from build123d import *

# Parameters (mm, degrees)
F0_W = 19.05
F0_H = 38.1
F2_R = 6.35


with BuildPart() as f1:
    # F0 (on Front) → F1 (revolve)
    with BuildSketch(Plane.XZ):
        with BuildLine():
            Line((-38.1, 100.1140274882), (-69.85, 100.1140274882))
            ThreePointArc((-69.85, 100.1140274882), (-78.8302561211, 96.3942836093), (-82.55, 87.4140274882))
            Line((-82.55, 87.4140274882), (-82.55, -115.7859725118))
            ThreePointArc((-82.55, -115.7859725118), (-78.8302561211, -124.7662286328), (-69.85, -128.4859725118))
            Line((-69.85, -128.4859725118), (-19.05, -128.4859725118))
            Line((-19.05, -128.4859725118), (-19.05, 100.1140274882))
            Line((-19.05, 100.1140274882), (-38.1, 100.1140274882))
        make_face()
        with Locations((-28.575, 119.1640274882)):
            Rectangle(F0_W, F0_H)
    revolve(axis=Axis((-19.05, 0, 11.2281292677), (0, 0, -1)))

    # F2
    f2_edges = [f1.edges().sort_by_distance(p)[0] for p in [
        (0, 0, 100.114027),
        (0, 0, 138.214027),
    ]]
    fillet(f2_edges, radius=F2_R)


solid = f1.part
Geometry check sheet. Reference: the model listing, model coordinates, mm. A direction names the side the tool comes from. Round coordinates to 2 decimals unless told otherwise and drop trailing zeros. Order: outer loops, then holes, each group sorted by start corner. A loop starts at its lowest first (then second) coordinate and runs counter-clockwise, first axis right, second up. Notation, with made-up numbers: M 63,14.25 L 110,14.25 A14 cw 110,30.25 Z; hole C 38,11 d8. An arc over 180 degrees is marked long. Write each question's results on one line, items separated by ' | '. Start each with the question number.
1. Cross-section at B-B on x = -19.05. Record the boundary of the cut face in (y, z), plus the area to 3 significant figures.
2. Set-up check for faces 1 (the face through (-3.93, -11.59, 119.34)), 2 (the face through (-19, 0, 138.214)): record each of +Z, -Z, +X, -X, +Y, -Y from which the full face is reachable in a straight line by a thin tool's end or side.
3. Cross-section at A-A on y = 0. Record the boundary of the cut face in (x, z).
4. Material ranges on L1, parallel to Y at x = -74, z = 42.5; L2, parallel to Y at x = -20, z = -16; L3, parallel to Z at x = -33, y = -42.5, recorded low to high. Write a range as from..to.
5. Cross-section at C-C on z = 75. Record the boundary of the cut face in (x, y), plus the area to 3 significant figures.
6. Go/stop test with flat-tipped pins: P1, Ø6, axis at y = -31, z = -5.5, coming from the -X side; P2, Ø2, axis at x = 8, z = -73.5, coming from the +Y side; P3, Ø4, axis at y = -10.5, z = -70, coming from the -X side. Record where each tip stops, or that it passes through.
Resolved:
1) outline: M -63.5,-115.79 A12.7 ccw -50.8,-128.49 L 50.8,-128.49 A12.7 ccw 63.5,-115.79 L 63.5,87.41 A12.7 ccw 50.8,100.11 L 25.4,100.11 A6.35 cw 19.05,106.46 L 19.05,131.86 A6.35 ccw 12.7,138.21 L -12.7,138.21 A6.35 ccw -19.05,131.86 L -19.05,106.46 A6.35 cw -25.4,100.11 L -50.8,100.11 A12.7 ccw -63.5,87.41 Z | area: 30,300 mm2
2) face 1: +Z | face 2: +Z, +X, -X, +Y, -Y
3) outline: M -82.55,-115.79 A12.7 ccw -69.85,-128.49 L 31.75,-128.49 A12.7 ccw 44.45,-115.79 L 44.45,87.41 A12.7 ccw 31.75,100.11 L 6.35,100.11 A6.35 cw 0,106.46 L 0,131.86 A6.35 ccw -6.35,138.21 L -31.75,138.21 A6.35 ccw -38.1,131.86 L -38.1,106.46 A6.35 cw -44.45,100.11 L -69.85,100.11 A12.7 ccw -82.55,87.41 Z
4) L1: -31.82..31.82 | L2: -63.49..63.49 | L3: -128.49..100.11
5) outline: C -19.05,0 d127 | area: 12,700 mm2
6) P1: x = -76.04 | P2: y = 57.91 | P3: x = -81.98
